```python
from build123d import *

# Parameters (mm, degrees)
SKETCH1_W           = 6.477
SKETCH1_H           = 6.477
BOSS_EXTRUDE1_DEPTH = 76.2
FILLET1_R           = 3.175
FILLET2_R           = 0.79375
SKETCH2_R           = 0.396875
CUT_EXTRUDE1_DEPTH  = 95.254215992
FILLET3_R           = 0.79375


with BuildPart() as part:
    # Sketch1 → Boss-Extrude1 (new body)
    with BuildSketch(Plane.XY):
        Polygon((-9.525, 0), (0, 0), (0, 9.525), (-7.714580181, 9.525), (-1.5875, 20.701), (42.8625, 20.701), (48.989580181, 9.525), (41.275, 9.525), (41.275, 0), (50.8, 0), (50.8, 9.525), (43.80259593, 22.2885), (-2.52759593, 22.2885), (-9.525, 9.525), align=None)
        with Locations((-4.7625, 4.7625)):
            Rectangle(SKETCH1_W, SKETCH1_H, mode=Mode.SUBTRACT)
        with Locations((46.0375, 4.7625)):
            Rectangle(SKETCH1_W, SKETCH1_H, mode=Mode.SUBTRACT)
    extrude(amount=BOSS_EXTRUDE1_DEPTH)

    # Fillet1
    fillet1_edges = [part.edges().sort_by_distance(p)[0] for p in [
        (-2.52759593, 22.2885, 38.1),
        (43.80259593, 22.2885, 38.1),
        (48.989580181, 9.525, 38.1),
        (42.8625, 20.701, 38.1),
        (-1.5875, 20.701, 38.1),
        (-7.714580181, 9.525, 38.1),
    ]]
    fillet(fillet1_edges, radius=FILLET1_R)

    # Fillet2
    fillet2_edges = [part.edges().sort_by_distance(p)[0] for p in [
        (0, 0, 38.1),
        (-9.525, 0, 38.1),
        (-9.525, 9.525, 38.1),
        (50.8, 9.525, 38.1),
        (50.8, 0, 38.1),
        (41.275, 0, 38.1),
        (41.275, 9.525, 38.1),
        (0, 9.525, 38.1),
    ]]
    fillet(fillet2_edges, radius=FILLET2_R)

    # Sketch2 → Cut-Extrude1 (cut, through all)
    with BuildSketch(Plane.XY.offset(76.2)):
        with Locations((-8.001, 8.001)):
            Circle(SKETCH2_R)
        with Locations((-1.524, 8.001)):
            Circle(SKETCH2_R)
        with Locations((-1.524, 1.524)):
            Circle(SKETCH2_R)
        with Locations((-8.001, 1.524)):
            Circle(SKETCH2_R)
        with Locations((42.799, 8.001)):
            Circle(SKETCH2_R)
        with Locations((42.799, 1.524)):
            Circle(SKETCH2_R)
        with Locations((49.276, 1.524)):
            Circle(SKETCH2_R)
        with Locations((49.276, 8.001)):
            Circle(SKETCH2_R)
    extrude(amount=-CUT_EXTRUDE1_DEPTH, mode=Mode.SUBTRACT)

    # Fillet3
    fillet3_edges = [part.edges().sort_by_distance(p)[0] for p in [
        (48.879125, 8.001, 38.1),
        (43.195875, 8.001, 38.1),
        (49.276, 1.920875, 38.1),
        (43.195875, 1.524, 38.1),
        (-1.920875, 1.524, 38.1),
        (-7.604125, 1.524, 38.1),
        (-8.001, 7.604125, 38.1),
        (-1.920875, 8.001, 38.1),
        (42.799, 7.604125, 38.1),
        (-8.001, 1.920875, 38.1),
        (-1.524, 1.920875, 38.1),
        (-1.524, 7.604125, 38.1),
        (42.799, 1.920875, 38.1),
        (48.879125, 1.524, 38.1),
        (49.276, 7.604125, 38.1),
        (-7.604125, 8.001, 38.1),
    ]]
    fillet(fillet3_edges, radius=FILLET3_R)


solid = part.part
```
Could you check a few things on this model? Use its own coordinates, in mm. A direction names the side the tool comes from. Give positions to 0.01 mm unless a question says otherwise; leave off trailing zeros. Order: outer loops, then holes, each group sorted by start corner. A loop starts at its lowest first (then second) coordinate and runs counter-clockwise, first axis right, second up.
Q1. I'm going to push flat-ended pins straight in: P1, Ø1.2, axis at x = -1.5, z = 50.5, coming from the +Y side; P2, Ø12, axis at x = 25, z = 53.5, coming from the -Y side; P3, Ø5, axis at x = 45, z = 34.5, coming from the +Y side; P4, Ø12, axis at x = 2.5, z = 16.5, coming from the -Y side. Where does each tip first touch, or does it pass through?
Q2. Suppose I cut it at D-D, the plane z = 65. Count the separate pieces of the cut face and the enclosed holes in it, and give its area (3 significant figures).
Q3. We'd pull the mould along X, two halves only. Please class faces 1 (the flat face through (20, 21, 76.2)), 2 (the flat face through (-6.387, 15.248, 37.567)), 3 (the cylindrical face through (46.38, 11.12, 38.63)): +X half, -X half, draft (parallel to the pull), parting line (faces both ways), or undercut.
Q4. Suppose I cut it at B-B, the plane y = 10.75. Write out the boundary of the cut face in (x, z), and give its area (3 significant figures).
Q5. If I drill on line 1 along X through (y, z) = (5.75, 49.5) (3 decimals); line 2 along X through (y, z) = (7.5, 6) (3 decimals); line 3 along Y through (x, z) = (13.5, 33), over which ranges is the centre line in solid material (lowest first)?
Q6. Suppose I cut it at C-C, the plane x = 34. Write out the boundary of the cut face in (y, z), and give its area (3 significant figures).
Q7. For faces 4 (the flat face through (-9.525, 5, 38)), 5 (the cylindrical face through (-1.346, 20.246, 38.633)), 6 (the flat face through (41.275, 5, 38)), which set-ups out of +Z, -Z, +X, -X, +Y, -Y let a thin tool reach every point of the face, with its end or its side?
Q8. Suppose I cut it at A-A, the plane y = 4. Write out the boundary of the cut face in (x, z) (3 decimals), and give its area (3 significant figures).
Solution:
1. P1: stops at y = 22.28
1. P2: stops at y = 20.7
1. P3: stops at y = 22.24
1. P4: stops at y = 0
2. separate pieces: 1
2. enclosed holes: 2
2. area: 222 mm2
3. face 1: draft
3. face 2: -X half
3. face 3: undercut
4. outline: (-8.85, 0) - (-4.86, 0) - (-4.86, 76.2) - (-8.85, 76.2) - close; (46.13, 0) - (50.13, 0) - (50.13, 76.2) - (46.13, 76.2) - close
4. area: 609 mm2
5. line 1: x = -9.525 to -8.001, -1.524 to 0, 41.275 to 42.799, 49.276 to 50.8
5. line 2: x = -9.525 to -8.101, -1.424 to 0, 41.275 to 42.699, 49.376 to 50.8
5. line 3: y = 20.7 to 22.29
6. outline: (20.7, 0) - (22.29, 0) - (22.29, 76.2) - (20.7, 76.2) - close
6. area: 121 mm2
7. face 4: +Z, -Z, -X, +Y, -Y
7. face 5: +Z, -Z
7. face 6: +Z, -Z, -Y
8. outline: (-9.525, 0) - (-8.001, 0) - (-8.001, 76.2) - (-9.525, 76.2) - close; (-1.524, 0) - (0, 0) - (0, 76.2) - (-1.524, 76.2) - close; (41.275, 0) - (42.799, 0) - (42.799, 76.2) - (41.275, 76.2) - close; (49.276, 0) - (50.8, 0) - (50.8, 76.2) - (49.276, 76.2) - close
8. area: 465 mm2
